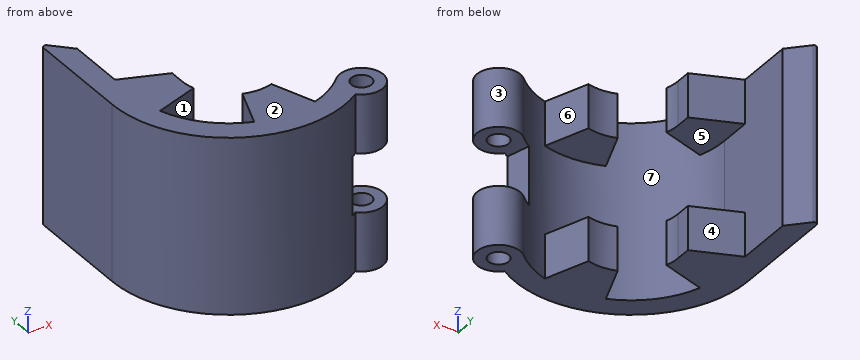
from build123d import *

# Parameters (mm, degrees)
SKETCH_1_R          = 1.75
EXTRUDE_1_DEPTH     = 15
EXTRUDE_START       = 15
EXTRUDE_2_DEPTH     = 7.5
EXTRUDE_START_2     = -7.5
EXTRUDE_3_DEPTH     = 7.5
SKETCH_1_5_R        = 1.75
CUT_EXTRUDE_2_DEPTH = 5


with BuildPart() as part:
    # Эскиз1 → Бобышка-Вытянуть1 (new, symmetric)
    with BuildSketch(Plane.XY):
        with BuildLine():
            Line((-15.95, 15.707106781), (-15.95, 0))
            ThreePointArc((-15.95, 0), (-6.103800746, -14.735878544), (11.27835316, -11.27835316))
            ThreePointArc((11.27835316, -11.27835316), (17.594576586, -13.917676686), (11.245989359, -16.478174151))
            ThreePointArc((11.245989359, -16.478174151), (-9.317859526, -17.640294608), (-19.95, 0))
            Line((-19.95, 0), (-19.95, 18.5))
            ThreePointArc((-19.95, 18.5), (-19.641341716, 18.961939766), (-19.096446609, 18.853553391))
            Line((-19.096446609, 18.853553391), (-15.95, 15.707106781))
        make_face()
        with Locations((13.89464825, -13.89464825)):
            Circle(SKETCH_1_R, mode=Mode.SUBTRACT)
    extrude(amount=EXTRUDE_1_DEPTH, both=True)

    # Эскиз1<3> → Бобышка-Вытянуть2 (add)
    with BuildSketch(Plane.XY.offset(EXTRUDE_START)):
        with BuildLine():
            ThreePointArc((-7.599342077, -2.5), (-7.899200485, -1.265950905), (-8, 0))
            Line((-8, 0), (-8, 2.645827558))
            Line((-8, 2.645827558), (-15.95, 5.539390921))
            Line((-15.95, 5.539390921), (-15.95, 0))
            ThreePointArc((-15.95, 0), (-15.728899355, -2.646549654), (-15.071727264, -5.219725787))
            Line((-15.071727264, -5.219725787), (-7.599342077, -2.5))
        make_face()
        with BuildLine():
            Line((-2.5, -7.599342077), (-5.219725787, -15.071727264))
            ThreePointArc((-5.219725787, -15.071727264), (0, -15.95), (5.219725787, -15.071727264))
            Line((5.219725787, -15.071727264), (2.5, -7.599342077))
            ThreePointArc((2.5, -7.599342077), (0, -8), (-2.5, -7.599342077))
        make_face()
    extrude(amount=-EXTRUDE_2_DEPTH)

    # Эскиз1<4> → Бобышка-Вытянуть3 (add)
    with BuildSketch(Plane.XY.offset(EXTRUDE_START_2)):
        with BuildLine():
            ThreePointArc((-7.599342077, -2.5), (-7.899200485, -1.265950905), (-8, 0))
            Line((-8, 0), (-8, 2.645827558))
            Line((-8, 2.645827558), (-15.95, 5.539390921))
            Line((-15.95, 5.539390921), (-15.95, 0))
            ThreePointArc((-15.95, 0), (-15.728899355, -2.646549654), (-15.071727264, -5.219725787))
            Line((-15.071727264, -5.219725787), (-7.599342077, -2.5))
        make_face()
        with BuildLine():
            Line((-2.5, -7.599342077), (-5.219725787, -15.071727264))
            ThreePointArc((-5.219725787, -15.071727264), (0, -15.95), (5.219725787, -15.071727264))
            Line((5.219725787, -15.071727264), (2.5, -7.599342077))
            ThreePointArc((2.5, -7.599342077), (0, -8), (-2.5, -7.599342077))
        make_face()
    extrude(amount=-EXTRUDE_3_DEPTH)

    # Эскиз1<5> → Вырез-Вытянуть2 (cut, symmetric)
    with BuildSketch(Plane.XY):
        with BuildLine():
            ThreePointArc((11.27835316, -11.27835316), (10.318427509, -12.162752721), (9.289403961, -12.965703762))
            Line((9.289403961, -12.965703762), (10.394358671, -17.028206242))
            ThreePointArc((10.394358671, -17.028206242), (10.823668488, -16.758600791), (11.245989359, -16.478174151))
            ThreePointArc((11.245989359, -16.478174151), (17.594576586, -13.917676686), (11.27835316, -11.27835316))
        make_face()
        with Locations((13.89464825, -13.89464825)):
            Circle(SKETCH_1_5_R, mode=Mode.SUBTRACT)
    extrude(amount=CUT_EXTRUDE_2_DEPTH, both=True, mode=Mode.SUBTRACT)


solid = part.part
Read the model definition and answer for the solid it produces. Units are mm, in the model's axes. Face numbers are marked on the shaded views. A direction names the side the tool comes from. Round coordinates to 2 decimals unless told otherwise and drop trailing zeros. Write each loop counter-clockwise with the first axis right and the second up, starting at its lowest first coordinate (ties: lowest second). Pieces come first, ordered by that corner, then holes. Notation, with made-up numbers: (65.5, -26) - (78.5, -26) arc R24 ccw to (78.5, 13) - close; hole circle Ø5 at (-16, 19). An arc over 180 degrees is marked (long way). Use a Markdown table: item, result.
(1) The mould has two halves that part along Y. Classify the marked faces 1, 2, 3 and 4: released by +Y, released by -Y, zero draft, split by the parting line, or undercut.
Reported:
| item | result |
|---|---|
| face 1 | undercut |
| face 2 | zero draft |
| face 3 | split by the parting line |
| face 4 | released by +Y |
(2) The part is cut by section B-B (x = 13.5). Write down the section's boundary in (y, z).
Reported:
| item | result |
|---|---|
| outline | (-17.57, -15) - (-15.6, -15) - (-15.6, -5) - (-17.57, -5) - close; (-17.57, 5) - (-15.6, 5) - (-15.6, 15) - (-17.57, 15) - close; (-12.19, -15) - (-10.22, -15) - (-10.22, -5) - (-12.19, -5) - close; (-12.19, 5) - (-10.22, 5) - (-10.22, 15) - (-12.19, 15) - close |
(3) Straight lines are drawn through the part: line 1 along X through (y, z) = (-13, 11.5); line 2 along Z through (x, y) = (16, -13); line 3 along Z through (x, y) = (1, -10). For each, find the intervals that lie inside material, in ascending order. Write a range as [from, to].
Reported:
| item | result |
|---|---|
| line 1 | [-15.13, -9.24], [-4.47, 4.47], [9.24, 12.39], [15.4, 17.48] |
| line 2 | [-15, -5], [5, 15] |
| line 3 | [-15, -7.5], [7.5, 15] |
(4) The part is cut by section C-C (z = 11.25). Write down the section's boundary in (x, y), then the cut area to 3 significant figures.
Reported:
| item | result |
|---|---|
| outline | (-19.95, 0) arc R19.95 ccw to (11.25, -16.48) arc R3.7 ccw (long way) to (11.28, -11.28) arc R15.95 cw to (5.22, -15.07) - (2.5, -7.6) arc R8 cw to (-2.5, -7.6) - (-5.22, -15.07) arc R15.95 cw to (-15.07, -5.22) - (-7.6, -2.5) arc R8 cw to (-8, 0) - (-8, 2.65) - (-15.95, 5.54) - (-15.95, 15.71) - (-19.1, 18.85) arc R0.5 ccw to (-19.95, 18.5) - close; hole circle Ø3.5 at (13.89, -13.89) |
| area | 388 mm2 |
(5) Which of the six approach directions +Z, -Z, +X, -X, +Y, -Y give full straight-line access (tool end or side, diameter ignored) to the marked faces 5, 6 and 7?
Reported:
| item | result |
|---|---|
| face 5 | +X, +Y |
| face 6 | +Z, -Z, +Y |
| face 7 | none |
(6) The part is cut by section D-D (x = 0.5). Write down the section's boundary in (y, z).
Reported:
| item | result |
|---|---|
| outline | (-19.94, -15) - (-7.98, -15) - (-7.98, -7.5) - (-15.94, -7.5) - (-15.94, 7.5) - (-7.98, 7.5) - (-7.98, 15) - (-19.94, 15) - close |
(7) Each of these flat-tipped pins is pushed along its axis until it touches: pin 1 Ø6 at (x, z) = (2.5, -3.5) entering from +Y; pin 2 Ø10 at (x, z) = (4, -7) entering from -Y; pin 3 Ø8 at (x, z) = (1, 3) entering from +Y; pin 4 Ø2 at (y, z) = (1, -9.5) entering from +X. Where does it stop, or does it pass through?
Reported:
| item | result |
|---|---|
| pin 1 | y = -14.97 |
| pin 2 | y = -19.95 |
| pin 3 | y = -15.15 |
| pin 4 | x = -8 |
(8) The part is cut by section A-A (z = 4). Write down the section's boundary in (x, y), then the cut area to 3 significant figures.
Reported:
| item | result |
|---|---|
| outline | (-19.95, 0) arc R19.95 ccw to (10.39, -17.03) - (9.29, -12.97) arc R15.95 cw to (-15.95, 0) - (-15.95, 15.71) - (-19.1, 18.85) arc R0.5 ccw to (-19.95, 18.5) - close |
| area | 225 mm2 |
